Input: part model. Units: mm. Frame: model coordinates. Round coordinates to 2 decimals unless told otherwise and drop trailing zeros. Write each loop counter-clockwise with the first axis right and the second up, starting at its lowest first coordinate (ties: lowest second). Pieces come first, ordered by that corner, then holes. Notation, with made-up numbers: (61.5, 88) -> (92.5, 88) arc R5 cw to (92.5, 95) -> close; hole circle Ø6 at (53.25, 68.5). An arc over 180 degrees is marked (long way). Use CSV: the item, a comma, the result in double quotes.
```python
from build123d import *

# Parameters (mm, degrees)
SKETCH1_R           = 1.778
BOSS_EXTRUDE1_DEPTH = 6.35


with BuildPart() as part:
    # Sketch1 → Boss-Extrude1 (new body)
    with BuildSketch(Plane(origin=(0, 6.35, 0), x_dir=(1, 0, 0), z_dir=(0, 1, 0))):
        with BuildLine():
            Line((78.232, 4.7625), (-78.232, 4.7625))
            ThreePointArc((-78.232, 4.7625), (-82.9945, 0), (-78.232, -4.7625))
            Line((-78.232, -4.7625), (78.232, -4.7625))
            ThreePointArc((78.232, -4.7625), (82.9945, 0), (78.232, 4.7625))
        make_face()
        with Locations((78.232, 0)):
            Circle(SKETCH1_R, mode=Mode.SUBTRACT)
        with Locations((68.453, 0)):
            Circle(SKETCH1_R, mode=Mode.SUBTRACT)
        with Locations((58.674, 0)):
            Circle(SKETCH1_R, mode=Mode.SUBTRACT)
        with Locations((48.895, 0)):
            Circle(SKETCH1_R, mode=Mode.SUBTRACT)
        with Locations((39.116, 0)):
            Circle(SKETCH1_R, mode=Mode.SUBTRACT)
        with Locations((29.337, 0)):
            Circle(SKETCH1_R, mode=Mode.SUBTRACT)
        with Locations((19.558, 0)):
            Circle(SKETCH1_R, mode=Mode.SUBTRACT)
        with Locations((9.779, 0)):
            Circle(SKETCH1_R, mode=Mode.SUBTRACT)
        Circle(SKETCH1_R, mode=Mode.SUBTRACT)
        with Locations((-9.779, 0)):
            Circle(SKETCH1_R, mode=Mode.SUBTRACT)
        with Locations((-19.558, 0)):
            Circle(SKETCH1_R, mode=Mode.SUBTRACT)
        with Locations((-29.337, 0)):
            Circle(SKETCH1_R, mode=Mode.SUBTRACT)
        with Locations((-39.116, 0)):
            Circle(SKETCH1_R, mode=Mode.SUBTRACT)
        with Locations((-48.895, 0)):
            Circle(SKETCH1_R, mode=Mode.SUBTRACT)
        with Locations((-58.674, 0)):
            Circle(SKETCH1_R, mode=Mode.SUBTRACT)
        with Locations((-68.453, 0)):
            Circle(SKETCH1_R, mode=Mode.SUBTRACT)
        with Locations((-78.232, 0)):
            Circle(SKETCH1_R, mode=Mode.SUBTRACT)
    extrude(amount=-BOSS_EXTRUDE1_DEPTH)


solid = part.part
```
Item 1: Pull-direction query (Z, two-part tool) for faces 1 (the face through (-1, 3, 4.762)), 2 (the face through (76.456, 3.219, -0.078)), 3 (the face through (82.993, 3.219, 0.105)); classes: +Z half, -Z half, draft (parallel to the pull), parting line (faces both ways), or undercut.
Worked answers:
face 1,"+Z half"
face 2,"undercut"
face 3,"parting line"
Item 2: Section query B-B on y = 5. Give the number of separate pieces and of enclosed holes in the cut face, plus the area to 3 significant figures.
Worked answers:
separate pieces,"1"
enclosed holes,"17"
area,"1,390 mm²"
Item 3: First-contact query: pin 1 Ø3 at (x, z) = (9.779, 0) entering from +Y; pin 2 Ø1.5 at (y, z) = (5, 3.5) entering from +X. Flat tips, straight axial feed; report the tip coordinate or a pass-through.
Worked answers:
pin 1,"passes through"
pin 2,"stops at x = 82.12"
Item 4: Section query A-A on x = 0. Return the cut outline in (y, z).
Worked answers:
outline,"(0, -4.76) -> (6.35, -4.76) -> (6.35, -1.78) -> (0, -1.78) -> close; (0, 1.78) -> (6.35, 1.78) -> (6.35, 4.76) -> (0, 4.76) -> close"
Item 5: Line query: line 1 (X direction, y = 2.5, z = -4); line 2 (X direction, y = 1.75, z = 2.75). Output: solid intervals per line, ascending.
Worked answers:
line 1,"x = -80.82 to 80.82"
line 2,"x = -82.12 to 82.12"
